from build123d import *

# Parameters (mm, degrees)
CROQUIS1_R              = 1.75
CROQUIS1_R_2            = 4.75
SALIENTE_EXTRUIR1_DEPTH = 2
REDONDEO1_R             = 1.5
CROQUIS2_W              = 9.5
CROQUIS2_H              = 5
SALIENTE_EXTRUIR2_DEPTH = 7.5
CROQUIS3_R              = 0.9
CORTAR_EXTRUIR1_DEPTH   = 5
SALIENTE_EXTRUIR3_DEPTH = 2
REDONDEO2_R             = 2
REDONDEO3_R             = 2
CROQUIS5_W              = 1.35
CROQUIS5_H              = 3
SALIENTE_EXTRUIR4_DEPTH = 1


with BuildPart() as part:
    # Croquis1 → Saliente-Extruir1 (new body)
    with BuildSketch(Plane.XY):
        with BuildLine():
            Line((10, -24), (8, -24))
            Line((8, -24), (-8, -24))
            Line((-8, -24), (-10, -24))
            ThreePointArc((-10, -24), (-11.149780948, -22.933215846), (-12.621352058, -22.390534425))
            ThreePointArc((-12.621352058, -22.390534425), (-15.586404832, -20.210444436), (-15.515491876, -16.530865429))
            ThreePointArc((-15.515491876, -16.530865429), (-15.043435032, -14.307276752), (-15.859153127, -12.185534953))
            ThreePointArc((-15.859153127, -12.185534953), (-20, 0), (-15.859153127, 12.185534953))
            ThreePointArc((-15.859153127, 12.185534953), (-15.043435032, 14.307276752), (-15.515491876, 16.530865429))
            ThreePointArc((-15.515491876, 16.530865429), (-15.667833806, 20.035019732), (-13, 22.312072261))
            ThreePointArc((-13, 22.312072261), (-10.83772234, 23.735565864), (-10, 26.185055607))
            Line((-10, 26.185055607), (-10, 28))
            Line((-10, 28), (10, 28))
            Line((10, 28), (10, 26.185055607))
            ThreePointArc((10, 26.185055607), (10.83772234, 23.735565864), (13, 22.312072261))
            ThreePointArc((13, 22.312072261), (15.667833806, 20.035019732), (15.515491876, 16.530865429))
            ThreePointArc((15.515491876, 16.530865429), (15.043435032, 14.307276752), (15.859153127, 12.185534953))
            ThreePointArc((15.859153127, 12.185534953), (20, 0), (15.859153127, -12.185534953))
            ThreePointArc((15.859153127, -12.185534953), (15.043435032, -14.307276752), (15.515491876, -16.530865429))
            ThreePointArc((15.515491876, -16.530865429), (15.586404832, -20.210444436), (12.621352058, -22.390534425))
            ThreePointArc((12.621352058, -22.390534425), (11.149780948, -22.933215846), (10, -24))
        make_face()
        with Locations((-12, -18.439088915)):
            Circle(CROQUIS1_R, mode=Mode.SUBTRACT)
        with Locations((12, -18.439088915)):
            Circle(CROQUIS1_R, mode=Mode.SUBTRACT)
        with Locations((12, 18.439088915)):
            Circle(CROQUIS1_R, mode=Mode.SUBTRACT)
        with Locations((-12, 18.439088915)):
            Circle(CROQUIS1_R, mode=Mode.SUBTRACT)
        Circle(CROQUIS1_R_2, mode=Mode.SUBTRACT)
    extrude(amount=SALIENTE_EXTRUIR1_DEPTH)

    # Redondeo1
    redondeo1_edges = [part.edges().sort_by_distance(p)[0] for p in [
        (-4.75, 0, 2),
    ]]
    fillet(redondeo1_edges, radius=REDONDEO1_R)

    # Croquis2 → Saliente-Extruir2 (add, symmetric)
    with BuildSketch(Plane(origin=(0, 0, 0), x_dir=(0, 0, -1), z_dir=(1, 0, 0))):
        with Locations((4.75, 19.4)):
            Rectangle(CROQUIS2_W, CROQUIS2_H)
        with Locations((4.75, -9.1)):
            Rectangle(CROQUIS2_W, CROQUIS2_H)
    extrude(amount=SALIENTE_EXTRUIR2_DEPTH, both=True)

    # Croquis3 → Cortar-Extruir1 (cut)
    with BuildSketch(Plane(origin=(0, 0, -9.5), x_dir=(-1, 0, 0), z_dir=(0, 0, -1))):
        with Locations((0, -8.75)):
            Circle(CROQUIS3_R)
        with Locations((0, 19.05)):
            Circle(CROQUIS3_R)
    extrude(amount=-CORTAR_EXTRUIR1_DEPTH, mode=Mode.SUBTRACT)

    # Croquis4 → Saliente-Extruir3 (add)
    with BuildSketch(Plane.ZY.offset(7.5)):
        Polygon((-9.5, -11.6), (0, -16.029922752), (0, -11.6), align=None)
        Polygon((-9.5, 21.9), (0, 21.9), (0, 26.329922752), align=None)
    saliente_extruir3 = extrude(amount=-SALIENTE_EXTRUIR3_DEPTH)

    # Simetría1: Saliente-Extruir3 across plane
    add(saliente_extruir3.mirror(Plane(origin=(0, 0, 0), x_dir=(0, 0, 1), z_dir=(1, 0, 0))))

    # Redondeo2
    redondeo2_edges = [part.edges().sort_by_distance(p)[0] for p in [
        (-5.5, -11.6, -4.75),
        (-5.5, 21.9, -4.75),
        (5.5, -11.6, -4.75),
        (5.5, 21.9, -4.75),
    ]]
    fillet(redondeo2_edges, radius=REDONDEO2_R)

    # Redondeo3
    redondeo3_edges = [part.edges().sort_by_distance(p)[0] for p in [
        (-7.5, 16.9, -4.75),
        (7.5, 16.9, -4.75),
        (-7.5, -6.6, -4.75),
        (7.5, -6.6, -4.75),
    ]]
    fillet(redondeo3_edges, radius=REDONDEO3_R)

    # Croquis5 → Saliente-Extruir4 (add)
    with BuildSketch(Plane(origin=(0, 0, -9.5), x_dir=(-1, 0, 0), z_dir=(0, 0, -1))):
        with Locations((-6.825, -10.1)):
            Rectangle(CROQUIS5_W, CROQUIS5_H)
        with Locations((6.825, -10.1)):
            Rectangle(CROQUIS5_W, CROQUIS5_H)
        with Locations((6.825, 20.4)):
            Rectangle(CROQUIS5_W, CROQUIS5_H)
        with Locations((-6.825, 20.4)):
            Rectangle(CROQUIS5_W, CROQUIS5_H)
    extrude(amount=SALIENTE_EXTRUIR4_DEPTH)


solid = part.part
Read the model definition and answer for the solid it produces. Units are mm, in the model's axes. A direction names the side the tool comes from. Coordinates: 2 decimals unless noted, no trailing zeros. Loops run counter-clockwise (first coordinate to the right, second up) from the corner with the lowest first, then second, coordinate; pieces in that order, holes last.
Q1. The part is cut by section D-D on y = -14.5. Write down the section's boundary in (x, z), and give its area (3 significant figures).
Q2. Which of the six approach directions +Z, -Z, +X, -X, +Y, -Y give full straight-line access (tool end or side, diameter ignored) to faces 5 (the face through (0, -6.6, -5)), 6 (the face through (6.9, -7.17, -4.82)), 7 (the face through (-6.93, -7.2, -4.82)), 8 (the face through (5.5, -14, -1))?
Q3. The mould has two halves that part along Y. Classify faces 1 (the face through (0, -24, 1)), 2 (the face through (5, 2, 0)), 3 (the face through (6, 24, -5)), 4 (the face through (0, 8, 2)): +Y half, -Y half, draft (parallel to the pull), parting line (faces both ways), or undercut.
Q4. The part is cut by section B-B on z = -8. Write down the section's boundary in (x, y).
Q5. The part is cut by section C-C on x = 12. Write down the section's boundary in (y, z).
Q6. Each of these flat-tipped pins is pushed along its axis until it touches: pin 1 Ø1.1 at (x, z) = (-7, -10) entering from -Y; pin 2 Ø0.5 at (x, z) = (-6.5, -10) entering from +Y; pin 3 Ø4 at (x, y) = (-12, -18.44) entering from -Z; pin 4 Ø2 at (x, y) = (-12, 18.44) entering from +Z. Where does it stop, or does it pass through?
Q7. The part is cut by section A-A on y = 0. Write down the section's boundary in (x, z), and give its area (3 significant figures).
Q8. Consider probe 1 along Y at (x, z) = (2, -3.75); probe 2 along Y at (x, z) = (12, 1.4); probe 3 along X at (y, z) = (24, -0.5). Determine where each line is inside the solid, lowest interval first.
Results below:
1. outline: (-15.03, 0) - (-7.5, 0) - (-7.5, -3.28) - (-5.5, -3.28) - (-5.5, 0) - (5.5, 0) - (5.5, -3.28) - (7.5, -3.28) - (7.5, 0) - (15.03, 0) - (15.03, 2) - (-15.03, 2) - close
1. area: 73.3 mm2
2. face 5: -Z, +X, -X
2. face 6: -Z, +X
2. face 7: -Z, -X
2. face 8: -Z, -Y
3. face 1: -Y half
3. face 2: undercut
3. face 3: +Y half
3. face 4: draft
4. outline: (-7.5, -12.3) - (-5.02, -12.3) arc R2 cw to (-3.5, -11.6) - (3.5, -11.6) arc R2 cw to (5.02, -12.3) - (7.5, -12.3) - (7.5, -8.6) arc R2 ccw to (5.5, -6.6) - (-5.5, -6.6) arc R2 ccw to (-7.5, -8.6) - close; (-7.5, 18.9) arc R2 ccw to (-5.5, 16.9) - (5.5, 16.9) arc R2 ccw to (7.5, 18.9) - (7.5, 22.6) - (5.02, 22.6) arc R2 cw to (3.5, 21.9) - (-3.5, 21.9) arc R2 cw to (-5.02, 22.6) - (-7.5, 22.6) - close; hole circle Ø1.8 at (0, -8.75); hole circle Ø1.8 at (0, 19.05)
5. outline: (-22.54, 0) - (-20.19, 0) - (-20.19, 2) - (-22.54, 2) - close; (-16.69, 0) - (16.69, 0) - (16.69, 2) - (-16.69, 2) - close; (20.19, 0) - (22.72, 0) - (22.72, 2) - (20.19, 2) - close
6. pin 1: stops at y = -11.62
6. pin 2: stops at y = 21.9
6. pin 3: stops at z = 0
6. pin 4: passes through
7. outline: (-20, 0) - (-4.75, 0) - (-4.75, 0.5) arc R1.5 ccw to (-6.25, 2) - (-20, 2) - close; (4.75, 0) - (20, 0) - (20, 2) - (6.25, 2) arc R1.5 ccw to (4.75, 0.5) - close
7. area: 60.0 mm2
8. probe 1: y = -11.6 to -6.6, 16.9 to 21.9
8. probe 2: y = -22.54 to -20.19, -16.69 to 16.69, 20.19 to 22.72
8. probe 3: x = -7.5 to -5.5, 5.5 to 7.5
